Autodesk Inventor part; units mm, degrees
ref_plane "Work Plane8" through (0, 0, 20) normal (0, 0, 1) x (1, 0, 0)
ref_plane "YZ Plane" through (0, 0, 0) normal (1, 0, 0) x (0, 1, 0)
ref_plane "XZ Plane" through (0, 0, 0) normal (0, 1, 0) x (-1, 0, 0)
sketch "Sketch1" plane through (0, 0, 0) normal (0, 0, 1) x (1, 0, 0)
  circle A0 centre (0, 0) radius 59.2469 construction
  line L0 (0, 0) -> (59.2469, 0)
  line L1 (0, 0) -> (59.2469, 4.025)
  line L2 (59.2469, 0) -> (59.2469, 4.025)
  circle A1 centre (0, 0) radius 75
  point P0 (56.8, 0)
  dimension "d56" = 59.2469
  dimension "d57" = 4.025
  dimension "d400" = 75
  dimension "d495" = 2.5
  dimension "d496" = 8
  dimension "d531" = 5.5
  dimension "d532" = 5.5
  dimension "d533" = 5.5
  dimension "d537" = 24.5
  dimension "d538" = 3
  dimension "d543" = 5.5
  dimension "d549" = 3
  dimension "d550" = 3
  dimension "d567" = 5.5
  dimension "d568" = 5.5
sketch "Sketch7" plane through (0, 0, 0) normal (0, 1, 0) x (-1, 0, 0)
  line L0 (0, 0) -> (0, 61.9844)
  line L1 (0, 0) -> (-59.2469, 0) construction
  line L2 (0, 61.9844) -> (-59.2469, 0) construction
  line L3 (0, 61.9844) -> (-64.8494, 0) construction
  line L4 (0, 61.9844) -> (-58.9939, -5.5968) construction
  line L5 (0, 0) -> (0, -61.9844)
  line L6 (0, -61.9844) -> (-59.2469, 0) construction
  line L7 (0, -61.9844) -> (-64.8494, 0) construction
  line L8 (0, -61.9844) -> (-58.9939, 5.5968) construction
  line L9 (-58.9939, 5.5968) -> (-64.8494, 0) construction
  line L10 (-54.1083, 0) -> (-62.8579, -8.363) construction
  line L11 (-54.1083, 0) -> (-38.773, -14.6579) construction
  line L12 (0, -94.3812) -> (0, 132.3969)
  line L13 (-75, -5.9919) -> (-75, 6.008)
  line L14 (105, 0) -> (-105, 0)
  line L15 (-62.0481, 2.6775) -> (-56.4456, -2.6775) construction
  line L16 (-56.4456, 2.6775) -> (-62.0481, -2.6775) construction
  line L17 (-26.151, -15.9303) -> (-40.3783, -15.9303) construction
  line L18 (-40.3783, -15.9303) -> (-40.3783, -12.7539) construction
  line L19 (-40.3783, -12.7539) -> (-26.151, -12.7539) construction
  line L20 (-26.151, -12.7539) -> (-26.151, -15.9303) construction
  point P0 (-75, 0)
  dimension "Roller_Side_difference" = -0.0002
  dimension "d90" = 61.9844
  dimension "d201" = 75
  dimension "d343" = 92.587
  dimension "d344" = 92.588
  dimension "d367" = 8.1
sketch "Roller1" plane through (0, 0, 0) normal (0, 1, 0) x (-1, 0, 0)
  line L0 (0, 61.9844) -> (-58.9939, -5.5968) construction
  line L1 (0, 61.9844) -> (-64.8494, 0) construction
  line L2 (-54.1083, 0) -> (-38.773, -14.6579) construction
  line L3 (0, -61.9844) -> (-64.8494, 0) construction
  line L4 (-54.0606, 0.0927) -> (-58.9462, -5.5041)
  line L5 (-58.9462, -5.5041) -> (-64.7589, 0.0519)
  line L6 (-64.7589, 0.0519) -> (-59.3884, 5.1851)
  line L7 (-59.3884, 5.1851) -> (-54.0606, 0.0927)
  line L8 (-56.0019, 1.9482) -> (-61.1299, -3.4168)
  line L9 (-61.8526, -2.7261) -> (-56.7246, 2.639)
  point P0 (0, 0)
  dimension "d345" = 0.025
  dimension "d346" = 0.025
  dimension "d347" = 0.1
  dimension "d348" = 0.1
  dimension "d349" = 272.588
  dimension "d350" = 272.587
  dimension "d617" = 0.9997
sketch "Roller2" plane through (0, 0, 0) normal (0, 1, 0) x (-1, 0, 0)
  line L0 (0, -61.9844) -> (-58.9939, 5.5968) construction
  line L1 (-54.1083, 0) -> (-62.8579, -8.363) construction
  line L2 (0, -61.9844) -> (-64.8494, 0) construction
  line L3 (0, 61.9844) -> (-64.8494, 0) construction
  line L4 (-58.9956, 5.5606) -> (-54.1429, 0.0016)
  line L5 (-54.1429, 0.0016) -> (-59.4789, -5.0987)
  line L6 (-59.4789, -5.0987) -> (-64.8132, 0)
  line L7 (-64.8132, 0) -> (-58.9956, 5.5606)
  line L8 (-61.9044, 2.7803) -> (-56.8109, -2.5486)
  line L9 (-61.1815, 3.4713) -> (-56.088, -1.8576)
  point P0 (0, 0)
  dimension "d351" = 0.025
  dimension "d352" = 0.025
  dimension "d354" = 0.025
  dimension "d355" = 92.587
  dimension "d356" = 92.588
  dimension "d370" = 0.025
  dimension "d371" = 1
sketch "Sketch22" plane through (0, 0, 0) normal (0, 1, 0) x (-1, 0, 0)
  line L0 (-31.756, 8.0215) -> (-17.5287, 8.0215) construction
  line L1 (-17.5287, 8.0215) -> (-17.5287, 4.8451) construction
  line L2 (-17.5287, 4.8451) -> (-31.756, 4.8451) construction
  line L3 (-31.756, 4.8451) -> (-31.756, 8.0215) construction
  point P0 (0, 0)
  dimension "Roller_Side_difference" = -0.0002
sketch "Sketch2" plane through (0, 0, 0) normal (0, 1, 0) x (-1, 0, 0)
  line L0 (0, 0) -> (0, 59.2469) construction
  line L1 (0, 0) -> (-59.2469, 0)
  line L2 (0, 0) -> (0, -59.2469)
  line L3 (0, -59.2469) -> (-59.2469, 0) construction
  line L4 (0, 59.2469) -> (-59.2469, 0) construction
  line L5 (-50.4879, 53.555) -> (0, 59.2469) construction
  line L6 (-29.7354, 7.189) -> (0, 59.2469) construction
  line L7 (-29.7354, 7.189) -> (0, -59.2469) construction
  line L8 (-48.8381, -26.254) -> (0, -59.2469) construction
  point P0 (-40.4258, 18.8211)
sketch "Sketch23" plane through (0, 0, 0) normal (0, 1, 0) x (-1, 0, 0)
  line L0 (0, -61.9844) -> (-58.9939, 5.5968) construction
  line L1 (0, -61.9844) -> (-64.8494, 0) construction
  line L2 (0, 61.9844) -> (-58.9939, -5.5968) construction
  line L3 (-58.9939, 5.5968) -> (-64.8494, 0) construction
  line L4 (0, 61.9844) -> (-64.8494, 0) construction
  line L5 (-58.9939, 5.5968) -> (-58.9939, -5.5968) construction
  line L6 (105, 0) -> (-105, 0)
  line L7 (-57.6514, 4.0968) -> (-54.1326, 0.0658)
  line L8 (-54.1326, -0.0658) -> (-57.6514, -4.0968)
  line L9 (-60.5995, 4.0968) -> (-64.81, 0.0723)
  line L10 (-64.81, -0.0723) -> (-60.5995, -4.0968)
  arc A0 (-64.81, 0.0723) -> (-64.81, -0.0723) centre (-64.7409, 0) ccw
  arc A1 (-54.1326, -0.0658) -> (-54.1326, 0.0658) centre (-54.2079, 0) ccw
  line L11 (-57.6514, 4.0968) -> (-57.6514, 5.5968)
  line L12 (-57.6514, 5.5968) -> (-25, 5.5968)
  line L13 (-25, 5.5968) -> (-25, -5.5968)
  line L14 (-25, -5.5968) -> (-57.6514, -5.5968)
  line L15 (-57.6514, -5.5968) -> (-57.6514, -4.0968)
  line L16 (-60.5995, 4.0968) -> (-60.5995, 5.5968)
  line L17 (-60.5995, 5.5968) -> (-75, 5.5968)
  line L18 (-75, 5.5968) -> (-75, -5.5968)
  line L19 (-60.5995, -4.0968) -> (-60.5995, -5.5968)
  line L20 (-60.5995, -5.5968) -> (-75, -5.5968)
  line L21 (-58.9939, 5.5968) -> (-58.9939, 5.5968)
  line L22 (-58.9939, -5.5968) -> (-58.9939, -5.5968)
  line L23 (0, -94.3812) -> (0, 132.3969)
  line L24 (-64.8856, 0) -> (-75, 0)
  point P0 (0, 0)
  point P1 (-54.0752, 0)
  point P2 (-64.8409, 0)
  point P3 (-75, 0)
  dimension "d378" = 90
  dimension "d379" = 0.1
  dimension "d380" = 0.025
  dimension "d381" = 0.025
  dimension "d382" = 0.025
  dimension "d383" = 0.025
  dimension "d384" = 11.1935
  dimension "d385" = 0
  dimension "d386" = 0
  dimension "d391" = 25
  dimension "d392" = 75
  dimension "d393" = 1.5
  dimension "d394" = 1.5
  dimension "d395" = 1.5
  dimension "d396" = 1.5
revolve "RevRoller1" [suppressed]
fillet "Fillet1" [suppressed]
sketch "Sketch48" plane through (56.7246, 0, 2.639) normal (-0.691, 0, 0.7229) x (0.7229, 0, 0.691)
  line L0 (-2.5, 0.25) -> (2.5, 0.25)
  line L1 (2.5, 0.25) -> (2.5, -0.25)
  line L2 (2.5, -0.25) -> (-2.5, -0.25)
  line L3 (-2.5, -0.25) -> (-2.5, 0.25)
  line L4 (-2.5, 0.25) -> (2.5, -0.25) construction
  line L5 (2.5, 0.25) -> (-2.5, -0.25) construction
  line L6 (-0.25, -2.5) -> (0.25, -2.5)
  line L7 (0.25, -2.5) -> (0.25, 2.5)
  line L8 (0.25, 2.5) -> (-0.25, 2.5)
  line L9 (-0.25, 2.5) -> (-0.25, -2.5)
  line L10 (-0.25, -2.5) -> (0.25, 2.5) construction
  line L11 (0.25, -2.5) -> (-0.25, 2.5) construction
  point P0 (-42.8293, 0)
  point P1 (0, 0)
  point P2 (-0.25, 0.25)
  point P3 (-0.25, -0.25)
  point P4 (0.25, -0.25)
  point P5 (0.25, 0.25)
  dimension "d621" = 5
  dimension "d622" = 0.5
  dimension "d623" = 0.5
  dimension "d624" = 5
extrude "Extrusion39" [suppressed]
sketch "Sketch40" plane through (0, 0, -5.231) normal (0, 0, -1) x (-1, 0, 0)
  circle A0 centre (53.5, 0) radius 2.75
  circle A1 centre (0, 0) radius 53.5
  point P0 (53.4293, 2.7491)
  point P1 (53.4293, -2.7491)
  dimension "d585" = 8
  dimension "d587" = 1.75
  dimension "d589" = 3
  dimension "d592" = 2
  dimension "d593" = 12
  dimension "d594" = 12
  dimension "d611" = 360
pattern_circular "Circular Pattern13" [suppressed]
feature "Move Body7" [suppressed]
revolve "Revolution13" [suppressed]
fillet "Fillet3" [suppressed]
pattern_circular "Circular Pattern14" [suppressed]
feature "Move Body6" [suppressed]
revolve "Revolution14" add sketch "Sketch23" angle 360 about axis through (0, 0, -10) along (0, 0, 1) contours A1 L7 L11 L12 L13 L6 | L6 L13 L14 L15 L8 A1
revolve "OuterRim_Top2" [suppressed]
revolve "OuterRim_Bottom2" [suppressed]
ref_plane "Work Plane8" through (0, 0, 20) normal (0, 0, 1) x (1, 0, 0)
sketch "Sketch49" plane through (0, 0, 20) normal (0, 0, 1) x (1, 0, 0)
  circle A0 centre (0, 0) radius 75
  circle A1 centre (0, 0) radius 60.5995
  circle A2 centre (0, 0) radius 57.6514
  circle A3 centre (0, 0) radius 25
  circle A4 centre (0, 0) radius 69
  circle A5 centre (0, 0) radius 36.75
  point P0 (0, 69)
  point P1 (0, 36.75)
  point P2 (-40.5572, 55.8222)
  dimension "d629" = 69
  dimension "d630" = 73.5
  dimension "d649" = 36
sketch "Sketch50" plane through (0, 0, 5.5968) normal (0, 0, 1) x (1, 0, 0)
  point P0 (0, 0)
  point P1 (0, 69)
sketch "Sketch51" plane through (0, 0, -5.5968) normal (0, 0, -1) x (-1, 0, 0)
  circle A0 centre (0, 0) radius 75
  circle A1 centre (0, 69) radius 2.75
  circle A2 centre (0, 69) radius 1.5
  circle A3 centre (-40.5572, 55.8222) radius 3.5
  circle A4 centre (-40.5572, 55.8222) radius 2
  dimension "d633" = 36
  dimension "d635" = 5.5
  dimension "d636" = 3
  dimension "d637" = 7
  dimension "d638" = 4
extrude "Extrusion40" [suppressed]
extrude "Extrusion41" [suppressed]
extrude "Extrusion42" [suppressed]
extrude "Extrusion43" [suppressed]
sketch "Sketch52" plane through (0, 0, 5.5968) normal (0, 0, 1) x (1, 0, 0)
  circle A0 centre (0, 69) radius 1.5
  circle A1 centre (-40.5572, 55.8222) radius 2
  line L0 (2.75, 67.4123) -> (0, 65.8246)
  line L1 (0, 65.8246) -> (-2.75, 67.4123)
  line L2 (-2.75, 67.4123) -> (-2.75, 70.5877)
  line L3 (-2.75, 70.5877) -> (0, 72.1754)
  line L4 (0, 72.1754) -> (2.75, 70.5877)
  line L5 (2.75, 70.5877) -> (2.75, 67.4123)
  circle A2 centre (0, 0) radius 75
  line L6 (-39.2656, 58.7231) -> (-37.3992, 56.1541)
  line L7 (-36.5379, 56.2446) -> (-38.1817, 52.5526)
  line L8 (-38.1817, 52.5526) -> (-42.201, 52.1301)
  line L9 (-42.201, 52.1301) -> (-44.5765, 55.3997)
  line L10 (-44.5765, 55.3997) -> (-42.9327, 59.0918)
  line L11 (-42.9327, 59.0918) -> (-38.9134, 59.5142)
  line L12 (-38.9134, 59.5142) -> (-36.5379, 56.2446)
  dimension "d651" = 3
  dimension "d652" = 4
  dimension "d655" = 36
  dimension "d657" = 7
  dimension "d658" = 5.5
extrude "Extrusion44" [suppressed]
extrude "Extrusion45" [suppressed]
extrude "Extrusion46" [suppressed]
extrude "Extrusion47" [suppressed]
pattern_circular "Circular Pattern32" [suppressed]
pattern_circular "Circular Pattern33" [suppressed]
sketch "Sketch57" plane through (0, 0, -5.5968) normal (0, 0, -1) x (-1, 0, 0)
  line L0 (-3.175, 39.925) -> (3.175, 39.925)
  line L1 (3.175, 39.925) -> (3.175, 33.575)
  line L2 (3.175, 33.575) -> (-3.175, 33.575)
  line L3 (-3.175, 33.575) -> (-3.175, 39.925)
  line L4 (-3.175, 39.925) -> (3.175, 33.575) construction
  line L5 (3.175, 39.925) -> (-3.175, 33.575) construction
  ellipse E0 centre (0, 36.75) end of major axis (6, 36.75) minor radius 6
  circle A0 centre (0, 36.75) radius 2.4
  point P0 (0, 0)
  dimension "d694" = 6.35
  dimension "d695" = 6.35
  dimension "d696" = 6
  dimension "d697" = 6
  dimension "d705" = 4.8
extrude "Extrusion50" cut sketch "Sketch57" against normal blind 11.194 contours A0
extrude "Extrusion51" cut sketch "Sketch57" against normal blind 8.194 contours L0 L1 L2 L3 | E0 | A0
pattern_circular "Circular Pattern34" count 6 over 360 about axis through (0, 0, -4.8468) along (0, 0, 1) of "Extrusion50", "Extrusion51"
ref_plane "Work Plane9" through (0, 0, -25) normal (0, 0, 1) x (1, 0, 0)
sketch "Sketch58" plane through (0, 0, -25) normal (0, 0, 1) x (1, 0, 0)
  circle A0 centre (0, 0) radius 78.9709
  line L0 (0, 0) -> (0, 88.7109)
  line L1 (0, 0) -> (29.2038, 108.9901)
  line L2 (0, 0) -> (-27.1115, 101.1815)
  point P0 (-20.4392, 76.28)
  point P1 (20.4392, 76.28)
  dimension "d707" = 15
  dimension "d708" = 15
extrude "Extrusion52" cut sketch "Sketch58" along normal through all contours A0 L2 L1
equation "\"Roller_Side_difference\" = -0.000942deg"
equation "\"Cycloid_Top_Plate_Fasner_Inner\" = 61.25"
equation "\"Cycloid_Top_Plate_Fasner_Outer\" = 85.75"
equation "\"Roller_Hole_Radius\" = 1"
equation "\"Distance_To_Bearing\" = 85.74529"
equation "\"d514\" = 0.2"
equation "\"Machine_Screw_4mm_Head_Dept\" = 4"
equation "\"Machine_Screw_4mm_Head_Diameter\" = 7"
equation "\"Machine_Screw_4mm_HexNut_Thickness\" = 3"
equation "\"Machine_Screw_4mm_HexNut_Width\" = 6.9"
equation "\"Machine_Screw_4mm_Length\" = 8"
equation "\"Fastner_4mm_Hex_Nut_Width\" = 7"
equation "\"Fastner_4mm_Screw_Diameter\" = 4"
equation "\"Fastner_4mm_Screw_Head_Diameter\" = 7"
equation "\"Fastner_4mm_Hex_Nut_Hole_Dept\" = 3.19352"
equation "\"Fastner_4mm_Screw_Head_Hole_Dept\" = 4"
properties part number "Sectio_Right_OuterBearing_TBS"
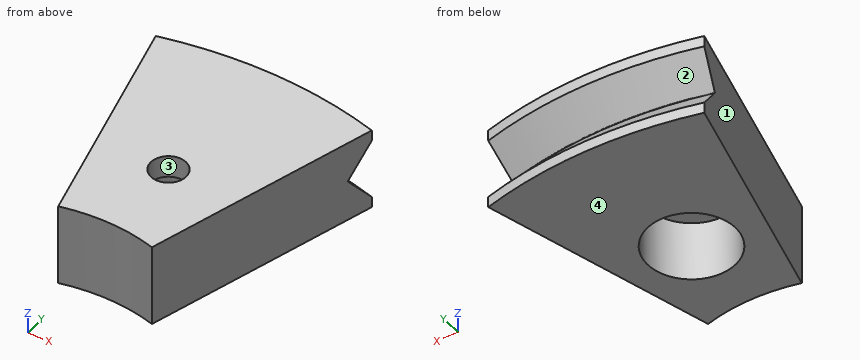
Could you check a few things on this model? Use its own coordinates, in mm. Face numbers are marked on the shaded views. Round coordinates to 2 decimals unless told otherwise and drop trailing zeros. Write each loop counter-clockwise with the first axis right and the second up, starting at its lowest first coordinate (ties: lowest second). Pieces come first, ordered by that corner, then holes. Notation, with made-up numbers: (-2.5, -20) -> (44.5, -20) arc R26 ccw to (44.5, 7) -> close; hole circle Ø9 at (48.5, 48). An arc over 180 degrees is marked (long way). Use a Markdown table: item, result.
1. For pin 1 Ø2 at (x, z) = (-4, 0.5) entering from -Y; pin 2 Ø3.5 at (x, y) = (-2, 38.5) entering from -Z; pin 3 Ø4 at (y, z) = (29, -4.5) entering from -X, each with a flat end and sliding along its axis, tell me the tip position at first contact or that it passes through.
Answer key:
| item | result |
|---|---|
| pin 1 | stops at y = 24.49 |
| pin 2 | stops at z = 2.6 |
| pin 3 | stops at x = -8.31 |
2. If we section it at B-B (y = 26): List the corners of the cut face in (x, z) for me, then the cut area to 3 significant figures.
Answer key:
| item | result |
|---|---|
| outline | (-6.97, -5.6) -> (6.97, -5.6) -> (6.97, 5.6) -> (-6.97, 5.6) -> close |
| area | 156 mm^2 |
3. We'd pull the mould along Y, two halves only. Please class the marked faces 1, 2, 3 and 4: +Y half, -Y half, draft (parallel to the pull), parting line (faces both ways), or undercut.
Answer key:
| item | result |
|---|---|
| face 1 | -Y half |
| face 2 | +Y half |
| face 3 | undercut |
| face 4 | draft |
4. Please list where these lines run through material, in increasing order: probe 1 along Y at (x, z) = (0, 4.5); probe 2 along Y at (x, z) = (3, -3.25); probe 3 along X at (y, z) = (31.5, -1.5).
Answer key:
| item | result |
|---|---|
| probe 1 | y = 25 to 34.35, 39.15 to 57.65 |
| probe 2 | y = 24.82 to 31.55, 41.95 to 56.83 |
| probe 3 | x = -8.44 to -2.9, 2.9 to 8.44 |
5. If we section it at A-A (z = 3.25): List the corners of the cut face in (x, y) for me, then the cut area to 3 significant figures.
Answer key:
| item | result |
|---|---|
| outline | (-14.73, 54.97) -> (-6.47, 24.15) arc R25 cw to (6.47, 24.15) -> (14.73, 54.97) arc R56.91 ccw to start; hole circle Ø4.8 at (0, 36.75) |
| area | 666 mm^2 |
